Could you check a few things on this drawing? It's one solid part, dimensions in mm from its lowest x, y, z. Round coordinates to 2 decimals unless told otherwise and drop trailing zeros. Loops run counter-clockwise (first coordinate to the right, second up) from the corner with the lowest first, then second, coordinate; pieces in that order, holes last.
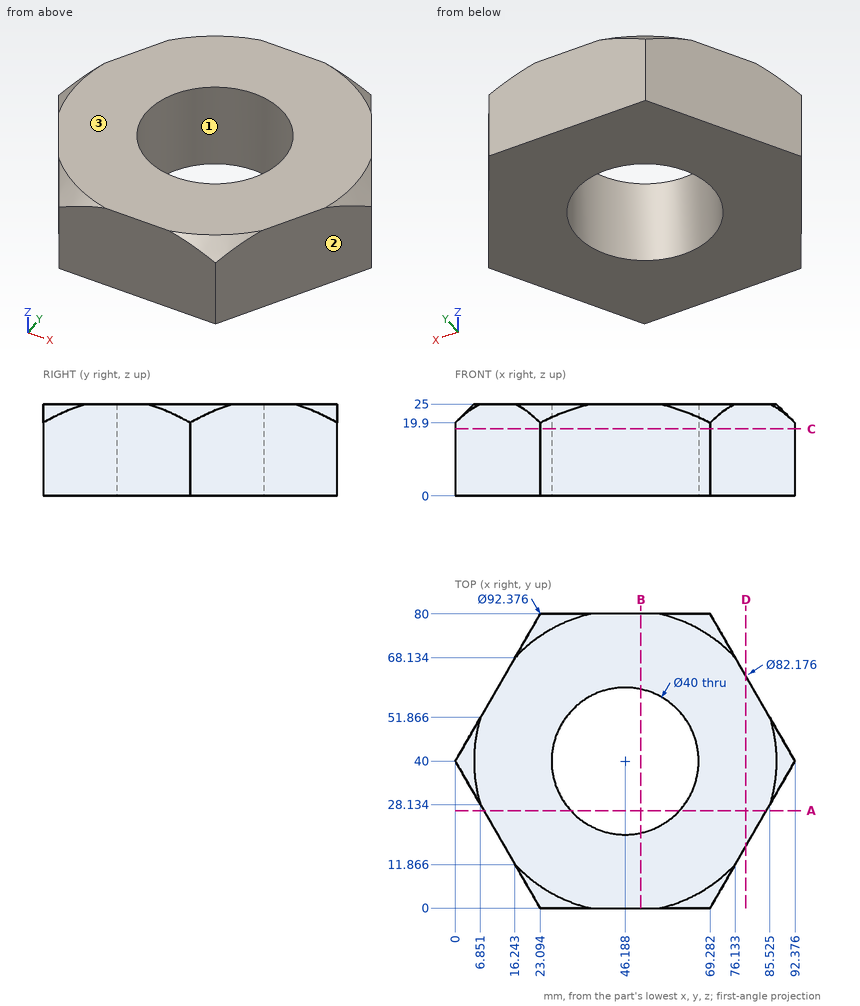
(1) Suppose I cut it at B-B (x = 50.5). Write out the boundary of the cut face in (y, z), then the cut area to 3 significant figures.
(2) For pin 1 (12 mm diameter, centred on y = 30.5, z = 7.5, fed in from +X) (1 decimal); pin 2 (1.5 mm diameter, centred on x = 80, z = 9.5, fed in from +Y) (1 decimal); pin 3 (1 mm diameter, centred on y = 37, z = 11, fed in from -X); pin 4 (12 mm diameter, centred on x = 77, y = 17.5, fed in from -Z), each with a flat end and sliding along its axis, tell me the tip position at first contact or that it passes through.
(3) We'd pull the mould along Y, two halves only. Please class the marked faces 1, 2 and 3: released by +Y, released by -Y, zero draft, split by the parting line, or undercut.
(4) If I drill on line 1 (X direction, y = 25.5, z = 14.75) (1 decimal); line 2 (Y direction, x = 56, z = 13.5); line 3 (X direction, y = 25, z = 11.75) (1 decimal), over which ranges is the centre line in solid material (lowest first)?
(5) Suppose I cut it at C-C (z = 18.25). Write out the boundary of the cut face in (x, y), then the cut area to 3 significant figures.
(6) Suppose I cut it at D-D (x = 79). Write out the boundary of the cut face in (y, z), then the cut area to 3 significant figures.
(7) Suppose I cut it at A-A (y = 26.5). Write out the boundary of the cut face in (x, z) (1 decimal).
Check result:
1. outline: (0, 0) - (20.47, 0) - (20.47, 25) - (0, 25) - close; (59.53, 0) - (80, 0) - (80, 25) - (59.53, 25) - close
1. area: 1,020 mm2
2. pin 1: stops at x = 90.4
2. pin 2: stops at y = 62.7
2. pin 3: stops at x = 1.44
2. pin 4: stops at z = 0
3. face 1: undercut
3. face 2: released by -Y
3. face 3: zero draft
4. line 1: x = 8.4 to 32.4, 60 to 84
4. line 2: y = 0 to 22.57, 57.43 to 80
4. line 3: x = 8.7 to 33, 59.4 to 83.7
5. outline: (0, 40) - (23.09, 0) - (69.28, 0) - (92.38, 40) - (69.28, 80) - (23.09, 80) - close; hole circle Ø40 at (46.19, 40)
5. area: 4,290 mm2
6. outline: (16.83, 0) - (63.17, 0) - (63.17, 25) - (16.83, 25) - close
6. area: 1,160 mm2
7. outline: (7.8, 0) - (31.4, 0) - (31.4, 25) - (7.8, 25) - close; (60.9, 0) - (84.6, 0) - (84.6, 25) - (60.9, 25) - close
